from build123d import *

# Parameters (mm, degrees)
SKETCH1_R           = 44.45
SKETCH1_W           = 63.5
SKETCH1_H           = 31.75
SKETCH1_H_2         = 44.45
BOSS_EXTRUDE1_DEPTH = 40.64
SKETCH1_3_R         = 44.45
SKETCH1_3_R_2       = 31.75
BOSS_EXTRUDE2_DEPTH = 76.2
SKETCH2_W           = 203.2
SKETCH2_H           = 12.7
BOSS_EXTRUDE3_DEPTH = 50.8
SKETCH3_R           = 5.842
CUT_EXTRUDE1_DEPTH  = 197.461447172


with BuildPart() as part:
    # Sketch1 → Boss-Extrude1 (new body)
    with BuildSketch(Plane(origin=(0, 0, 0), x_dir=(1, 0, 0), z_dir=(0, 1, 0))):
        Polygon((-22.225, 63.5), (-22.225, 165.1), (-47.625, 165.1), (-47.625, 63.5), (-47.625, -95.25), (-47.625, -158.75), (47.625, -158.75), (47.625, -95.25), (47.625, 63.5), (47.625, 165.1), (22.225, 165.1), (22.225, 63.5), align=None)
        with Locations(Location((0, 0, 0), (0, 0, 270))):
            Circle(SKETCH1_R, mode=Mode.SUBTRACT)
        with Locations((0, -127)):
            Rectangle(SKETCH1_W, SKETCH1_H, mode=Mode.SUBTRACT)
        with Locations((0, -69.85)):
            Rectangle(SKETCH1_W, SKETCH1_H_2, mode=Mode.SUBTRACT)
    extrude(amount=BOSS_EXTRUDE1_DEPTH)

    # Sketch1_3 → Boss-Extrude2 (add)
    with BuildSketch(Plane(origin=(0, 0, 0), x_dir=(1, 0, 0), z_dir=(0, 1, 0))):
        with Locations(Location((0, 0, 0), (0, 0, 270))):
            Circle(SKETCH1_3_R)
        with Locations(Location((0, 0, 0), (0, 0, 270))):
            Circle(SKETCH1_3_R_2, mode=Mode.SUBTRACT)
    extrude(amount=BOSS_EXTRUDE2_DEPTH)

    # Sketch2 → Boss-Extrude3 (add)
    with BuildSketch(Plane(origin=(47.625, 0, 0), x_dir=(0, 0, -1), z_dir=(1, 0, 0))):
        with Locations((0, 34.29)):
            Rectangle(SKETCH2_W, SKETCH2_H)
    extrude(amount=BOSS_EXTRUDE3_DEPTH)

    # Sketch3 → Cut-Extrude1 (cut, through all)
    with BuildSketch(Plane(origin=(0, 40.64, 0), x_dir=(1, 0, 0), z_dir=(0, 1, 0))):
        with Locations(Location((65.405, 76.2, 0), (0, 0, 270))):
            Circle(SKETCH3_R)
        with Locations(Location((65.405, -76.2, 0), (0, 0, 270))):
            Circle(SKETCH3_R)
        Polygon((47.625, 101.6), (85.725, 87.732734074), (85.725, 62.332734074), (47.625, 48.465468149), (47.625, -48.465468149), (85.725, -62.332734074), (85.725, -87.732734074), (47.625, -101.6), (98.425, -101.6), (98.425, 101.6), align=None)
    extrude(amount=-CUT_EXTRUDE1_DEPTH, mode=Mode.SUBTRACT)


solid = part.part
Input: part model. Units: mm. Frame: model coordinates. A direction names the side the tool comes from. Give positions to 0.01 mm unless a question says otherwise; leave off trailing zeros. Order: outer loops, then holes, each group sorted by start corner. A loop starts at its lowest first (then second) coordinate and runs counter-clockwise, first axis right, second up. Notation, with made-up numbers: (28, -26.75) - (78, -26.75) arc R15 cw to (78, -7.75) - close; hole circle Ø9 at (64.25, -10). An arc over 180 degrees is marked (long way). Write each question's results on one line, items separated by ' | '.
Item 1: Draft query along Z for faces 1 (the cylindrical face through (37.48, 58.17, 23.9)), 2 (the flat face through (22.225, 20, -115)), 3 (the flat face through (-31.75, 20, 127)). Return one class per face: released by +Z, released by -Z, zero draft, split by the parting line, or undercut.
A:
face 1: split by the parting line | face 2: zero draft | face 3: undercut
Item 2: Section B-B (x = 76). Return loops of the section in (y, z).
A:
outline: (27.94, -91.27) - (40.64, -91.27) - (40.64, -58.79) - (27.94, -58.79) - close; (27.94, 58.79) - (40.64, 58.79) - (40.64, 91.27) - (27.94, 91.27) - close
Item 3: Section C-C (y = 18). Return loops of the section in (x, z) (3 decimals).
A:
outline: (-47.625, -165.1) - (-22.225, -165.1) - (-22.225, -63.5) - (22.225, -63.5) - (22.225, -165.1) - (47.625, -165.1) - (47.625, 158.75) - (-47.625, 158.75) - close; hole circle Ø63.5 at (0, 0); hole (-31.75, 47.625) - (31.75, 47.625) - (31.75, 92.075) - (-31.75, 92.075) - close; hole (-31.75, 111.125) - (31.75, 111.125) - (31.75, 142.875) - (-31.75, 142.875) - close
Item 4: Material intervals for line 1 along X through (y, z) = (53.5, 0); line 2 along Z through (x, y) = (-13.5, 9) (3 decimals); line 3 along Z through (x, y) = (-25.5, 27) (3 decimals), sorted ascending.
A:
line 1: x = -44.45 to -31.75, 31.75 to 44.45 | line 2: z = -63.5 to -28.737, 28.737 to 47.625, 92.075 to 111.125, 142.875 to 158.75 | line 3: z = -165.1 to -18.916, 18.916 to 47.625, 92.075 to 111.125, 142.875 to 158.75
Item 5: Contact query for flat-ended pins moving along their axis: pin 1 Ø9.5 at (y, z) = (23.5, 123.5) entering from +X (3 decimals); pin 2 Ø20.5 at (x, y) = (5.5, 25.5) entering from -Z; pin 3 Ø5 at (x, y) = (32.5, 66) entering from +Z; pin 4 Ø10.5 at (x, z) = (65.405, -76.2) entering from -Y. Output: stop coordinate, or through.
A:
pin 1: stops at x = 47.625 | pin 2: stops at z = -63.5 | pin 3: stops at z = 32.8 | pin 4: passes through
Item 6: Section A-A (z = -76.2). Return loops of the section in (x, y) (3 decimals), and give its area (3 significant figures).
A:
outline: (-47.625, 0) - (-22.225, 0) - (-22.225, 40.64) - (-47.625, 40.64) - close; (22.225, 0) - (47.625, 0) - (47.625, 27.94) - (59.563, 27.94) - (59.563, 40.64) - (22.225, 40.64) - close; (71.247, 27.94) - (85.725, 27.94) - (85.725, 40.64) - (71.247, 40.64) - close | area: 2,400 mm^2
Item 7: Section D-D (z = -19.5). Return loops of the section in (x, y) (3 decimals), and give its area (3 significant figures).
A:
outline: (-47.625, 0) - (-25.056, 0) - (-25.056, 76.2) - (-39.944, 76.2) - (-39.944, 40.64) - (-47.625, 40.64) - close; (25.056, 0) - (47.625, 0) - (47.625, 40.64) - (39.944, 40.64) - (39.944, 76.2) - (25.056, 76.2) - close | area: 2,890 mm^2
Item 8: Access query for faces 4 (the flat face through (0, 20, 111.125)), 5 (the flat face through (62, 27.94, 70)), 6 (the flat face through (47.625, 20, -1)). Directions: +Z, -Z, +X, -X, +Y, -Y. A direction counts if a zero-diameter tool reaches every point of the face in a straight line with its end or side. Return the directions, or none.
A:
face 4: +Y, -Y | face 5: +Z, -Z, +X, -Y | face 6: +X, -Y
